Read the model definition and answer for the solid it produces. Units are mm, in the model's axes. A direction names the side the tool comes from. Coordinates: 2 decimals unless noted, no trailing zeros. Order: outer loops, then holes, each group sorted by start corner. A loop starts at its lowest first (then second) coordinate and runs counter-clockwise, first axis right, second up. Notation, with made-up numbers: M 39.25,56 L 68.25,56 A10 cw 68.25,66 Z; hole C -0.75,54 d10. An arc over 180 degrees is marked long. Put each result on its own line as item: value.
from build123d import *

# Parameters (mm, degrees)
SKETCH_1_W          = 23.9
SKETCH_1_H          = 32.9
EXTRUDE_1_DEPTH     = 3
SHELL_1_T           = -0.2
SKETCH_3_2_W        = 9
SKETCH_3_2_H        = 0.2
SKETCH_3_2_W_2      = 2
SKETCH_3_2_W_3      = 5
SKETCH_3_2_W_4      = 4
CUT_EXTRUDE_3_DEPTH = 2.8
SKETCH_3_W          = 3
SKETCH_3_H          = 0.2
SKETCH_3_W_2        = 0.2
SKETCH_3_H_2        = 3
EXTRUDE_2_DEPTH     = 3
FILLET_1_R          = 0.2
SKETCH_5_R          = 1
CUT_EXTRUDE_5_DEPTH = 7


with BuildPart() as part:
    # Sketch 1 → Extrude 1 (new body)
    with BuildSketch(Plane.XY):
        with Locations((11.8, 16.3)):
            Rectangle(SKETCH_1_W, SKETCH_1_H)
    extrude(amount=EXTRUDE_1_DEPTH)

    # Shell 1
    shell_1_openings = [part.faces().sort_by_distance(p)[0] for p in [
        (11.8, 16.3, 0),
    ]]
    offset(amount=SHELL_1_T, openings=shell_1_openings, kind=Kind.INTERSECTION)

    # Sketch 3_2 → Cut-Extrude 3 (cut)
    with BuildSketch(Plane(origin=(0, 0, 0), x_dir=(-1, 0, 0), z_dir=(0, 0, -1))):
        with Locations((-5.8, -0.05)):
            Rectangle(SKETCH_3_2_W, SKETCH_3_2_H)
        with Locations((-21.3, -0.05)):
            Rectangle(SKETCH_3_2_W_2, SKETCH_3_2_H)
        with Locations((-13.3, 32.65)):
            Rectangle(SKETCH_3_2_W_3, SKETCH_3_2_H)
        with Locations((-3.3, 32.65)):
            Rectangle(SKETCH_3_2_W_4, SKETCH_3_2_H)
    extrude(amount=-CUT_EXTRUDE_3_DEPTH, mode=Mode.SUBTRACT)

    # Sketch 3 → Extrude 2 (add)
    with BuildSketch(Plane(origin=(0, 0, 0), x_dir=(-1, 0, 0), z_dir=(0, 0, -1))):
        with Locations((-9.3, 32.65)):
            Rectangle(SKETCH_3_W, SKETCH_3_H)
        with Locations((0.05, 11.8)):
            Rectangle(SKETCH_3_W_2, SKETCH_3_H_2)
        with Locations((-23.65, 11.8)):
            Rectangle(SKETCH_3_W_2, SKETCH_3_H_2)
    extrude(amount=EXTRUDE_2_DEPTH)

    # Fillet 1
    fillet_1_edges = [part.edges().sort_by_distance(p)[0] for p in [
        (-0.05, 13.3, -3),
        (-0.05, 10.3, -3),
        (23.65, 13.3, -3),
        (23.65, 10.3, -3),
        (1.3, -0.05, 0),
        (10.3, -0.05, 0),
        (20.3, -0.05, 0),
        (22.3, -0.05, 0),
        (15.8, 32.65, 0),
        (1.3, 32.65, 0),
        (5.3, 32.65, 0),
        (7.8, 32.65, -3),
        (10.8, 32.65, -3),
    ]]
    fillet(fillet_1_edges, radius=FILLET_1_R)

    # Sketch 5 → Cut-Extrude 5 (cut, through all)
    with BuildSketch(Plane.XY.offset(3)):
        with Locations((11.8, 16.3)):
            Circle(SKETCH_5_R)
        with Locations((2.85, 29.75)):
            Circle(SKETCH_5_R)
        with Locations((2.85, 2.85)):
            Circle(SKETCH_5_R)
        with Locations((20.75, 2.85)):
            Circle(SKETCH_5_R)
        with Locations((20.75, 29.75)):
            Circle(SKETCH_5_R)
    extrude(amount=-CUT_EXTRUDE_5_DEPTH, mode=Mode.SUBTRACT)


solid = part.part
Q1. Find section D-D on y = 16.3. Write down the section's boundary in (x, z), plus the area to 3 significant figures.
Answers below:
outline: M -0.15,0 L 0.05,0 L 0.05,2.8 L 10.8,2.8 L 10.8,3 L -0.15,3 Z; M 12.8,2.8 L 23.55,2.8 L 23.55,0 L 23.75,0 L 23.75,3 L 12.8,3 Z
area: 5.50 mm^2
Q2. For a pull along Y with two mould halves and no side action, classify faces 3 (the face through (-0.15, 16, 1)), 4 (the face through (23.55, 16, 1)), 5 (the face through (12, -0.15, 1)), 6 (the face through (10, 32.75, 1)) as +Y half, -Y half, draft (parallel to the pull), parting line (faces both ways), or undercut.
Answers below:
face 3: draft
face 4: undercut
face 5: -Y half
face 6: +Y half
Q3. Find section B-B on y = 29.75. Write down the section's boundary in (x, z), plus the area to 3 significant figures.
Answers below:
outline: M -0.15,0 L 0.05,0 L 0.05,2.8 L 1.85,2.8 L 1.85,3 L -0.15,3 Z; M 3.85,2.8 L 19.75,2.8 L 19.75,3 L 3.85,3 Z; M 21.75,2.8 L 23.55,2.8 L 23.55,0 L 23.75,0 L 23.75,3 L 21.75,3 Z
area: 5.10 mm^2
Q4. Consider line 1 along Y through (x, z) = (2.85, 2.9); line 2 along X through (y, z) = (21, 1.25). Determine where each line is inside the solid, lowest interval first.
Answers below:
line 1: y = -0.15 to 1.85, 3.85 to 28.75, 30.75 to 32.75
line 2: x = -0.15 to 0.05, 23.55 to 23.75
Q5. A tool of negligible diameter and unlimited length cuts with its end or side. For faces 1 (the face through (23.75, 16, 1)), 2 (the face through (15, 0.05, 1)), from which of +Z, -Z, +X, -X, +Y, -Y can it reach the whole face along a straight path? Write none if from no direction.
Answers below:
face 1: +Z, -Z, +X, +Y, -Y
face 2: -Z
Q6. Find section A-A on x = 20.75. Write down the section's boundary in (y, z), plus the area to 3 significant figures.
Answers below:
outline: M -0.15,2.8 L 1.85,2.8 L 1.85,3 L -0.15,3 Z; M 3.85,2.8 L 28.75,2.8 L 28.75,3 L 3.85,3 Z; M 30.75,2.8 L 32.55,2.8 L 32.55,0 L 32.75,0 L 32.75,3 L 30.75,3 Z
area: 6.34 mm^2
Q7. Given pin 1 (10 mm diameter, centred on x = 14, y = 22, fed in from -Z); pin 2 (1.2 mm diameter, centred on x = 2.85, y = 2.85, fed in from -Z), each flat-ended and moving along its own axis, determine where each tip first touches the part or whether it passes through.
Answers below:
pin 1: stops at z = 2.8
pin 2: passes through
Q8. Find section C-C on z = 0.8. Write down the section's boundary in (x, y), plus the area to 3 significant figures.
Answers below:
outline: M -0.15,-0.15 L 1.3,-0.15 L 1.3,0.05 L 0.05,0.05 L 0.05,32.55 L 1.3,32.55 L 1.3,32.75 L -0.15,32.75 Z; M 5.3,32.55 L 10.8,32.55 L 10.8,32.75 L 5.3,32.75 Z; M 10.3,-0.15 L 20.3,-0.15 L 20.3,0.05 L 10.3,0.05 Z; M 15.8,32.55 L 23.55,32.55 L 23.55,0.05 L 22.3,0.05 L 22.3,-0.15 L 23.75,-0.15 L 23.75,32.75 L 15.8,32.75 Z
area: 18.6 mm^2
